The model under review builds one solid part; all positions refer to its coordinate system, in mm. A direction names the side the tool comes from. Round coordinates to 2 decimals unless told otherwise and drop trailing zeros. Order: outer loops, then holes, each group sorted by start corner. A loop starts at its lowest first (then second) coordinate and runs counter-clockwise, first axis right, second up. Notation, with made-up numbers: M 81.5,-12.5 L 90.5,-12.5 A14 ccw 90.5,0.5 Z; hole C -12.75,53 d8. An arc over 180 degrees is marked long. Answer as a JSON object with one key per item and string values. Group by question number.
1) For faces 4 (the flat face through (33.973, 5.705, 19.511)), 5 (the flat face through (22.882, 0, -1)), 6 (the flat face through (-20, 11, -26)), 7 (the conical face through (34.32, 22.67, 12.38)), list the 3-axis set-ups (+Z, -Z, +X, -X, +Y, -Y) from which the entire face can be reached by the end or side of a thin tool; tool diameter is ignored.
2) The part is to be moulded in two halves that separate along X. For faces 1 (the conical face through (34.45, 21.71, 12.41)), 2 (the conical face through (34.32, -22.67, 13.05)), 3 (the cylindrical face through (24.361, -26.702, 20.643)), say which applies: +X half, -X half, draft (parallel to the pull), parting line (faces both ways), or undercut.
3) To check wall thickness, follow line 1 (Z direction, x = 30.5, y = -12.5); line 2 (X direction, y = 14, z = -11); line 3 (Z direction, x = 4.5, y = 13). State the ranges of each line that lie inside material, in increasing order.
4) Consider section B-B, the plane x = -3. Write out the cut boundary in (y, z), then the cut area to 3 significant figures.
5) Consider section A-A, the plane z = -11. Write out the cut boundary in (x, y).
6) Insertion check: pin 1 Ø0.9 at (y, z) = (-21, 21.22) entering from +X; pin 2 Ø8 at (y, z) = (-20, -5) entering from +X; pin 3 Ø2.5 at (y, z) = (18, -26.5) entering from -X; pin 4 Ø4 at (x, y) = (0.38, 3.5) entering from +Z. Each pin has a flat end and moves straight along its axis. Give the tip position at first contact, or say it passes through.
```python
from build123d import *

# Parameters (mm, degrees)
EXTRUDE_1_DEPTH       = 27.5
SKETCH_3_R            = 0.75
CUT_EXTRUDE_3_DEPTH   = 3
REVOLVE_1_ANGLE       = 135
MIRROR_3_COPY_1_ANGLE = 135
MIRROR_3_COPY_2_ANGLE = 135
SKETCH_2_W            = 20
SKETCH_2_H            = 16.5
SKETCH_2_R            = 1.5
CUT_EXTRUDE_4_DEPTH   = 3
FILLET_1_R            = 5
FILLET_2_R            = 5


with BuildPart() as part:
    # 草图1 → 凸台-拉伸1 (new, symmetric)
    with BuildSketch(Plane(origin=(0, 0, 0), x_dir=(1, 0, 0), z_dir=(0, 1, 0))):
        Polygon((-30.117647059, 27.284313725), (25.882352941, 27.284313725), (25.882352941, -27.715686275), (22.882352941, -27.715686275), (22.882352941, 24.284313725), (-30.117647059, 24.284313725), align=None)
    extrude(amount=EXTRUDE_1_DEPTH, both=True)

    # 草图3 → 切除-拉伸3 (cut)
    with BuildSketch(Plane(origin=(25.882352941, 0, 0), x_dir=(0, 0, -1), z_dir=(1, 0, 0))):
        with BuildLine():
            Line((-12.715686275, 12.5), (-6.705278634, 6.48959236))
            ThreePointArc((-6.705278634, 6.48959236), (-4.862710248, 9.247190825), (-4.215686275, 12.5))
            ThreePointArc((-4.215686275, 12.5), (-6.705278634, 18.51040764), (-12.715686275, 21))
            Line((-12.715686275, 21), (-12.715686275, 12.5))
        make_face()
        with BuildLine():
            ThreePointArc((-12.715686275, 4), (-9.462877099, 4.647023974), (-6.705278634, 6.48959236))
            Line((-6.705278634, 6.48959236), (-12.715686275, 12.5))
            Line((-12.715686275, 12.5), (-12.715686275, 4))
        make_face()
        with BuildLine():
            Line((-12.715686275, 12.5), (-18.726093915, 6.48959236))
            ThreePointArc((-18.726093915, 6.48959236), (-15.96849545, 4.647023974), (-12.715686275, 4))
            Line((-12.715686275, 4), (-12.715686275, 12.5))
        make_face()
        with BuildLine():
            ThreePointArc((-12.715686275, 21), (-20.568662301, 15.752809175), (-18.726093915, 6.48959236))
            Line((-18.726093915, 6.48959236), (-12.715686275, 12.5))
            Line((-12.715686275, 12.5), (-12.715686275, 21))
        make_face()
        with BuildLine():
            Line((-12.715686275, 3), (-12.715686275, 0))
            Line((-12.715686275, 0), (-4.017201465, 0))
            ThreePointArc((-4.017201465, 0), (-4.536839235, 3.044356098), (-6.036908978, 5.743970558))
            ThreePointArc((-6.036908978, 5.743970558), (-9.105442495, 3.712728532), (-12.715686275, 3))
        make_face()
        with BuildLine():
            Line((-4.017201465, 0), (-12.715686275, 0))
            Line((-12.715686275, 0), (-12.715686275, -3))
            ThreePointArc((-12.715686275, -3), (-9.105442495, -3.712728532), (-6.036908978, -5.743970558))
            ThreePointArc((-6.036908978, -5.743970558), (-4.536839235, -3.044356098), (-4.017201465, 0))
        make_face()
        with BuildLine():
            Line((-19.394463571, 5.743970558), (-19.394463571, 0))
            Line((-19.394463571, 0), (-12.715686275, 0))
            Line((-12.715686275, 0), (-12.715686275, 3))
            ThreePointArc((-12.715686275, 3), (-16.325930054, 3.712728532), (-19.394463571, 5.743970558))
        make_face()
        with BuildLine():
            Line((-12.715686275, 0), (-19.394463571, 0))
            Line((-19.394463571, 0), (-19.394463571, -5.743970558))
            ThreePointArc((-19.394463571, -5.743970558), (-16.325930054, -3.712728532), (-12.715686275, -3))
            Line((-12.715686275, -3), (-12.715686275, 0))
        make_face()
        with BuildLine():
            Line((-6.705278634, -6.48959236), (-12.715686275, -12.5))
            Line((-12.715686275, -12.5), (-12.715686275, -21))
            ThreePointArc((-12.715686275, -21), (-6.705278634, -18.51040764), (-4.215686275, -12.5))
            ThreePointArc((-4.215686275, -12.5), (-4.862710248, -9.247190825), (-6.705278634, -6.48959236))
        make_face()
        with BuildLine():
            Line((-12.715686275, -4), (-12.715686275, -12.5))
            Line((-12.715686275, -12.5), (-6.705278634, -6.48959236))
            ThreePointArc((-6.705278634, -6.48959236), (-9.462877099, -4.647023974), (-12.715686275, -4))
        make_face()
        with BuildLine():
            ThreePointArc((-12.715686275, -4), (-15.96849545, -4.647023974), (-18.726093915, -6.48959236))
            Line((-18.726093915, -6.48959236), (-12.715686275, -12.5))
            Line((-12.715686275, -12.5), (-12.715686275, -4))
        make_face()
        with BuildLine():
            Line((-12.715686275, -12.5), (-18.726093915, -6.48959236))
            ThreePointArc((-18.726093915, -6.48959236), (-20.568662301, -15.752809175), (-12.715686275, -21))
            Line((-12.715686275, -21), (-12.715686275, -12.5))
        make_face()
        with Locations((-21.215686275, -21)):
            Circle(SKETCH_3_R)
        with Locations((-4.215686275, -21)):
            Circle(SKETCH_3_R)
        with Locations((-21.215686275, 21)):
            Circle(SKETCH_3_R)
        with Locations((-4.215686275, 21)):
            Circle(SKETCH_3_R)
        with BuildLine():
            ThreePointArc((-12.715686275, -3), (-16.325930054, -3.712728532), (-19.394463571, -5.743970558))
            Line((-19.394463571, -5.743970558), (-18.726093915, -6.48959236))
            ThreePointArc((-18.726093915, -6.48959236), (-15.96849545, -4.647023974), (-12.715686275, -4))
            ThreePointArc((-12.715686275, -4), (-9.462877099, -4.647023974), (-6.705278634, -6.48959236))
            Line((-6.705278634, -6.48959236), (-6.036908978, -5.743970558))
            ThreePointArc((-6.036908978, -5.743970558), (-9.105442495, -3.712728532), (-12.715686275, -3))
        make_face()
        with BuildLine():
            Line((-18.726093915, 6.48959236), (-19.394463571, 5.743970558))
            ThreePointArc((-19.394463571, 5.743970558), (-16.325930054, 3.712728532), (-12.715686275, 3))
            ThreePointArc((-12.715686275, 3), (-9.105442495, 3.712728532), (-6.036908978, 5.743970558))
            Line((-6.036908978, 5.743970558), (-6.705278634, 6.48959236))
            ThreePointArc((-6.705278634, 6.48959236), (-9.462877099, 4.647023974), (-12.715686275, 4))
            ThreePointArc((-12.715686275, 4), (-15.96849545, 4.647023974), (-18.726093915, 6.48959236))
        make_face()
        Polygon((-21.215686275, 27.5), (-23.783279652, 27.5), (-27.715686275, 27.5), (-27.715686275, 23.567593377), (-27.715686275, 20.249825378), (-27.715686275, 12.5), align=None)
        Polygon((-21.215686275, -27.5), (-27.715686275, -12.5), (-27.715686275, -20.249825378), (-27.715686275, -23.567593377), (-27.715686275, -27.5), (-23.783279652, -27.5), align=None)
    extrude(amount=-CUT_EXTRUDE_3_DEPTH, mode=Mode.SUBTRACT)

    # 草图5 → 旋转1 (revolve)
    with BuildSketch(Plane(origin=(0, 0, 12.715686275), x_dir=(0, -1, 0), z_dir=(0, 0, 1))):
        Polygon((-22, 25.882352941), (-21, 25.882352941), (-21, 31.882352941), (-23.5, 40.882352941), (-24.5, 40.882352941), (-22, 31.882352941), align=None)
    revolve_1 = revolve(axis=Axis((32.882352941, 12.5, 12.715686275), (-1, 0, 0)), revolution_arc=REVOLVE_1_ANGLE)

    # 镜向1: 旋转1 across plane
    add(revolve_1.mirror(Plane.ZX))

    # 镜向2: 旋转1 across plane
    add(revolve_1.mirror(Plane.XY.offset(12.715686275)))

    # 镜向3 copy 1 sketch → 镜向3 copy 1 (revolve)
    with BuildSketch(Plane.YX.offset(-12.715686275)):
        Polygon((-22, 25.882352941), (-21, 25.882352941), (-21, 31.882352941), (-23.5, 40.882352941), (-24.5, 40.882352941), (-22, 31.882352941), align=None)
    revolve(axis=Axis((32.882352941, -12.5, 12.715686275), (-1, 0, 0)), revolution_arc=MIRROR_3_COPY_1_ANGLE)

    # 镜向3 copy 2 sketch → 镜向3 copy 2 (revolve)
    with BuildSketch(Plane(origin=(0, 0, 12.715686275), x_dir=(0, -1, 0), z_dir=(0, 0, -1))):
        Polygon((-22, -25.882352941), (-21, -25.882352941), (-21, -31.882352941), (-23.5, -40.882352941), (-24.5, -40.882352941), (-22, -31.882352941), align=None)
    revolve(axis=Axis((32.882352941, 12.5, 12.715686275), (1, 0, 0)), revolution_arc=MIRROR_3_COPY_2_ANGLE)

    # 草图2 → 切除-拉伸4 (cut)
    with BuildSketch(Plane(origin=(0, 0, -27.284313725), x_dir=(-1, 0, 0), z_dir=(0, 0, -1))):
        with Locations((20.117647059, 19.25)):
            Rectangle(SKETCH_2_W, SKETCH_2_H)
        with Locations((-0.382352941, 3.5)):
            Circle(SKETCH_2_R)
        with Locations((19.617647059, 3.5)):
            Circle(SKETCH_2_R)
    extrude(amount=-CUT_EXTRUDE_4_DEPTH, mode=Mode.SUBTRACT)

    # 圆角1
    fillet_1_edges = [part.edges().sort_by_distance(p)[0] for p in [
        (22.882352941, 0, -24.284313725),
    ]]
    fillet(fillet_1_edges, radius=FILLET_1_R)

    # 圆角2
    fillet_2_edges = [part.edges().sort_by_distance(p)[0] for p in [
        (24.382352941, 12.5, 27.715686275),
        (24.382352941, 27.5, 21.215686275),
        (24.382352941, -12.5, 27.715686275),
        (24.382352941, -27.5, 21.215686275),
    ]]
    fillet(fillet_2_edges, radius=FILLET_2_R)


solid = part.part
```
Results list:
{
 "1": {"face 4": "+X", "face 5": "+Z, -X, +Y, -Y", "face 6": "+Z, -Z, -X, +Y", "face 7": "none"},
 "2": {"face 1": "+X half", "face 2": "undercut", "face 3": "draft"},
 "3": {"line 1": "3.22 to 4.22, 21.22 to 22.22", "line 2": "22.88 to 25.88", "line 3": "-27.28 to -24.28"},
 "4": {"outline": "M -27.5,-27.28 L 27.5,-27.28 L 27.5,-24.28 L -27.5,-24.28 Z", "area": "165 mm^2"},
 "5": {"outline": "M 22.88,-27.5 L 25.88,-27.5 L 25.88,27.5 L 22.88,27.5 Z"},
 "6": {"pin 1": "x = 40.88", "pin 2": "x = 25.88", "pin 3": "x = -10.12", "pin 4": "z = -24.28"}
}
